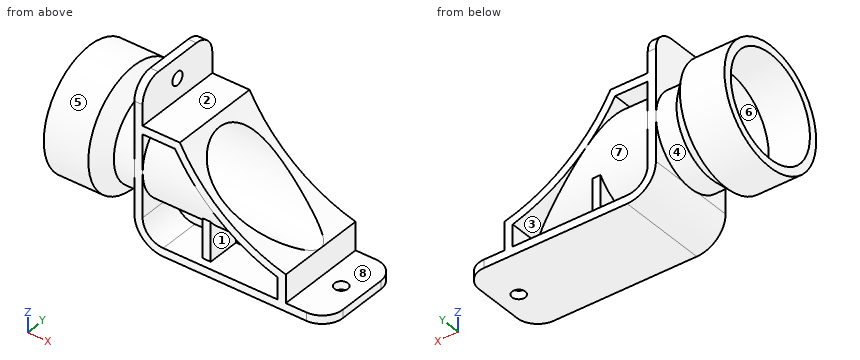
```python
from build123d import *
from build123d.topology import SkipClean

# Parameters (mm, degrees)
EXTRUDE_1_DEPTH                 = 11
EXTRUDE_1_DEPTH_BACK            = 11
EXTRUDE_6_REACH                 = 52.677
EXTRUDE_6_END_RADIUS            = 43
SKETCH_4_R                      = 11
EXTRUDE_6_DIRECTION_2_DEPTH     = 7
RIB_11_REACH                    = 52.677
SKETCH_7_WALL_W                 = 108.144859428
SKETCH_7_WALL_H                 = 2
RIB_12_REACH                    = 52.677
SKETCH_7_2_WALL_W               = 108.144859428
SKETCH_7_2_WALL_H               = 2
RIB_14_REACH                    = 40.859
SKETCH_8_WALL_W                 = 89.184699428
SKETCH_8_WALL_H                 = 2
CUT_EXTRUDE_1_REACH             = 52.677
CUT_EXTRUDE_1_END_RADIUS        = 41
SKETCH_9_R                      = 9
CUT_EXTRUDE_1_DIRECTION_2_DEPTH = 7
CUT_EXTRUDE_2_REACH             = 52.677
SKETCH_10_R                     = 1.6
CUT_EXTRUDE_3_REACH             = 60.998
SKETCH_11_R                     = 1.6
FILLET_1_R                      = 5


with BuildPart() as part:
    # 草图2 → 凸台-拉伸1 (new, two sides: drawn at the far end of the back side and taken through both)
    with BuildSketch(Plane(origin=(0, 0, 0), x_dir=(1, 0, 0), z_dir=(0, 1, 0)).offset(-EXTRUDE_1_DEPTH_BACK)):
        with BuildLine():
            Line((-2, 10.791694934), (-2, -21))
            Line((-2, -21), (0, -21))
            Line((0, -21), (0, -11))
            Line((0, -11), (9.04749367, -11))
            ThreePointArc((9.04749367, -11), (19.845447894, 1.668361044), (34.789686155, 9))
            Line((34.789686155, 9), (34.789686155, 15.791694934))
            Line((34.789686155, 15.791694934), (44.789686155, 15.791694934))
            Line((44.789686155, 15.791694934), (44.789686155, 17.791694934))
            Line((44.789686155, 17.791694934), (5, 17.791694934))
            ThreePointArc((5, 17.791694934), (0.050252532, 15.741442403), (-2, 10.791694934))
        make_face()
        with BuildLine():
            Line((0, 10.791694934), (0, -9))
            Line((0, -9), (7.881951948, -9))
            ThreePointArc((7.881951948, -9), (18.474626995, 3.135521358), (32.789686155, 10.521638371))
            Line((32.789686155, 10.521638371), (32.789686155, 15.791694934))
            Line((32.789686155, 15.791694934), (5, 15.791694934))
            ThreePointArc((5, 15.791694934), (1.464466094, 14.32722884), (0, 10.791694934))
        make_face(mode=Mode.SUBTRACT)
    extrude(amount=EXTRUDE_1_DEPTH + EXTRUDE_1_DEPTH_BACK)

    # 凸台-拉伸6: up to this cylinder (the profile starts outside it)
    extrude_6_end = Plane(origin=(45, 0, 30.708305066), z_dir=(0, 1, 0)) * Cylinder(EXTRUDE_6_END_RADIUS, 192.354, mode=Mode.PRIVATE)
    # 草图4 → 凸台-拉伸6 (add, up to the surface)
    with BuildSketch(Plane(origin=(0, 0, 0), x_dir=(0, 0, -1), z_dir=(1, 0, 0)), mode=Mode.PRIVATE) as extrude_6_sk1:
        Circle(SKETCH_4_R)
    extrude_6_tool1 = extrude(extrude_6_sk1.sketch, amount=EXTRUDE_6_REACH, mode=Mode.PRIVATE) - extrude_6_end
    add(extrude_6_tool1.solids().sort_by_distance((0, 0, 0))[0])

    # 草图4 → 凸台-拉伸6 direction 2 (add)
    with BuildSketch(Plane(origin=(0, 0, 0), x_dir=(0, 0, -1), z_dir=(1, 0, 0))):
        Circle(SKETCH_4_R)
    extrude(amount=-EXTRUDE_6_DIRECTION_2_DEPTH)

    # 草图7 wall → 筋11 (add, up to next)
    with BuildSketch(Plane(origin=(18.894843077, 0, -13.395847467), x_dir=(0, 0, 1), z_dir=(1, 0, 0)), mode=Mode.PRIVATE) as rib_11_sk1:
        Rectangle(SKETCH_7_WALL_W, SKETCH_7_WALL_H)
    rib_11_tool1 = extrude(rib_11_sk1.sketch, amount=-RIB_11_REACH, mode=Mode.PRIVATE) - part.part
    add(rib_11_tool1.solids().sort_by_distance((18.894843077, 0, -13.395847467))[0])

    # 草图7<2> wall → 筋12 (add, up to next)
    with BuildSketch(Plane(origin=(18.894843077, 0, -13.395847467), x_dir=(0, 0, 1), z_dir=(1, 0, 0)), mode=Mode.PRIVATE) as rib_12_sk1:
        Rectangle(SKETCH_7_2_WALL_W, SKETCH_7_2_WALL_H)
    rib_12_tool1 = extrude(rib_12_sk1.sketch, amount=RIB_12_REACH, mode=Mode.PRIVATE) - part.part
    add(rib_12_tool1.solids().sort_by_distance((18.894843077, 0, -13.395847467))[0])

    # 草图8 wall → 筋14 (add, up to next)
    with BuildSketch(Plane(origin=(14, 9, -11.058125127), x_dir=(0, 0, 1), z_dir=(0, -1, 0)), mode=Mode.PRIVATE) as rib_14_sk1:
        Rectangle(SKETCH_8_WALL_W, SKETCH_8_WALL_H)
    rib_14_tool1 = extrude(rib_14_sk1.sketch, amount=RIB_14_REACH, mode=Mode.PRIVATE) - part.part
    rib_14 = rib_14_tool1.solids().sort_by_distance((14, 9, -11.058125127))[0]
    add(rib_14)

    # 镜向1: 筋14 across plane
    add(rib_14.mirror(Plane.ZX))

    # 切除-拉伸1: up to this cylinder (the profile starts outside it)
    cut_extrude_1_end = Plane(origin=(45, 0, 30.708305066), z_dir=(0, 1, 0)) * Cylinder(CUT_EXTRUDE_1_END_RADIUS, 188.354, mode=Mode.PRIVATE)
    # 草图9 → 切除-拉伸1 (cut, up to the surface)
    with BuildSketch(Plane(origin=(0, 0, 0), x_dir=(0, 0, -1), z_dir=(1, 0, 0)), mode=Mode.PRIVATE) as cut_extrude_1_sk1:
        Circle(SKETCH_9_R)
    cut_extrude_1_tool1 = extrude(cut_extrude_1_sk1.sketch, amount=CUT_EXTRUDE_1_REACH, mode=Mode.PRIVATE) - cut_extrude_1_end
    add(cut_extrude_1_tool1.solids().sort_by_distance((0, 0, 0))[0], mode=Mode.SUBTRACT)

    # 草图9 → 切除-拉伸1 direction 2 (cut)
    with BuildSketch(Plane(origin=(0, 0, 0), x_dir=(0, 0, -1), z_dir=(1, 0, 0))):
        Circle(SKETCH_9_R)
    extrude(amount=-CUT_EXTRUDE_1_DIRECTION_2_DEPTH, mode=Mode.SUBTRACT)

    # 草图10 → 切除-拉伸2 (cut, up to next)
    with BuildSketch(Plane(origin=(0, 0, 0), x_dir=(0, 0, -1), z_dir=(1, 0, 0)), mode=Mode.PRIVATE) as cut_extrude_2_sk1:
        with Locations((-16, 0)):
            Circle(SKETCH_10_R)
    cut_extrude_2_tool1 = extrude(cut_extrude_2_sk1.sketch, amount=-CUT_EXTRUDE_2_REACH, mode=Mode.PRIVATE) & part.part
    add(cut_extrude_2_tool1.solids().sort_by_distance((0, 0, 16))[0], mode=Mode.SUBTRACT)

    # 草图11 → 切除-拉伸3 (cut, up to next)
    with BuildSketch(Plane.XY.offset(-15.791694934), mode=Mode.PRIVATE) as cut_extrude_3_sk1:
        with Locations((39.789686155, 0)):
            Circle(SKETCH_11_R)
    cut_extrude_3_tool1 = extrude(cut_extrude_3_sk1.sketch, amount=-CUT_EXTRUDE_3_REACH, mode=Mode.PRIVATE) & part.part
    add(cut_extrude_3_tool1.solids().sort_by_distance((39.789686, 0, -15.791695))[0], mode=Mode.SUBTRACT)

    # 圆角1
    fillet_1_edges = [part.edges().sort_by_distance(p)[0] for p in [
        (44.789686155, -11, -16.791694934),
        (-1, -11, 21),
        (-1, 11, 21),
        (44.789686155, 11, -16.791694934),
    ]]
    fillet(fillet_1_edges, radius=FILLET_1_R)

    # 草图14 → 旋转1 (revolve)
    with SkipClean():  # the faces are left unmerged after this step: merging them gives an invalid solid
        with BuildSketch(Plane.XY, mode=Mode.PRIVATE) as revolve_1_sk:
            Polygon((-10.5, 14.5), (-21.328427125, 14.5), (-21.328427125, 12.5), (-11.328427125, 12.5), (-7.828427125, 9), (-7, 9), (-7, 11), align=None)
        revolve(revolve_1_sk.sketch.rotate(Axis((-18.782404652, 0, 0), (1, 0, 0)), 90), axis=Axis((-18.782404652, 0, 0), (1, 0, 0)))


solid = part.part
```
Here's how the part is built. I have some questions about the finished solid (model axes, mm). Face numbers are marked on the shaded views. A direction names the side the tool comes from. Give positions to 0.01 mm unless a question says otherwise; leave off trailing zeros. Order: outer loops, then holes, each group sorted by start corner. A loop starts at its lowest first (then second) coordinate and runs counter-clockwise, first axis right, second up. Notation, with made-up numbers: M 11.25,-32.5 L 44.25,-32.5 A28 ccw 44.25,-6.5 Z; hole C 89,0 d7. An arc over 180 degrees is marked long. Use a Markdown table: item, result. Add a question column.
1. If we mould it in two halves opening along X, with no side actions, what happens to the marked faces 6, 7 and 8? For each: +X half, -X half, draft (parallel to the pull), parting line (faces both ways), or undercut.
2. For pin 1 Ø4 at (y, z) = (8.5, -13.5) entering from -X; pin 2 Ø5 at (y, z) = (-3.5, 18) entering from +X; pin 3 Ø1 at (x, z) = (9, 4.5) entering from -Y; pin 4 Ø6 at (x, z) = (23, -1) entering from -Y, each with a flat end and sliding along its axis, tell me the tip position at first contact or that it passes through.
3. I need wall thicknesses on probe 1 along Y at (x, z) = (-16.25, 0); probe 2 along X at (y, z) = (8.25, -13); probe 3 along Y at (x, z) = (12.5, 0). Which ranges of each line are inside material? Lowest first, please. Write a range as from..to.
4. Suppose I cut it at B-B (x = 37). List the corners of the cut face in (y, z) for me, and give its area (3 significant figures).
5. Suppose I cut it at A-A (y = 7.25). Give the number of separate pieces and of enclosed holes in the cut face, and give its area (3 significant figures).
6. On a 3-axis mill with a long thin cutter (end or side, diameter ignored), from which of +Z, -Z, +X, -X, +Y, -Y can I reach the whole of each face in a straight line? I mean the marked faces 1, 2, 3, 4 and 5. Say none if no direction works.
Results list:
| question | item | result |
|---|---|---|
| 1 | face 6 | -X half |
| 1 | face 7 | undercut |
| 1 | face 8 | draft |
| 2 | pin 1 | stops at x = -21.33 |
| 2 | pin 2 | stops at x = 0 |
| 2 | pin 3 | stops at y = -10.25 |
| 2 | pin 4 | stops at y = -11 |
| 3 | probe 1 | y = -14.5..-12.5, 12.5..14.5 |
| 3 | probe 2 | x = -1.64..0.51, 13..15, 32.79..34.79 |
| 3 | probe 3 | y = -11..-9, 9..11 |
| 4 | outline | M -11,-17.79 L 11,-17.79 L 11,-15.79 L -11,-15.79 Z |
| 4 | area | 44.0 mm² |
| 5 | separate pieces | 2 |
| 5 | enclosed holes | 3 |
| 5 | area | 423 mm² |
| 6 | face 1 | -Y |
| 6 | face 2 | +Z, +X, +Y, -Y |
| 6 | face 3 | +Y |
| 6 | face 4 | none |
| 6 | face 5 | -X |
